Can you work these out from the drawing? Everything is in mm from the part's minimum corner. A direction names the side the tool comes from. Coordinates: 2 decimals unless noted, no trailing zeros. Order: outer loops, then holes, each group sorted by start corner. A loop starts at its lowest first (then second) coordinate and runs counter-clockwise, first axis right, second up. Notation, with made-up numbers: (-25.75, 22) -> (23.25, 22) arc R21 cw to (23.25, 47) -> close; hole circle Ø11 at (-6, -28). An arc over 180 degrees is marked (long way). Answer in a Markdown table with one row per item.
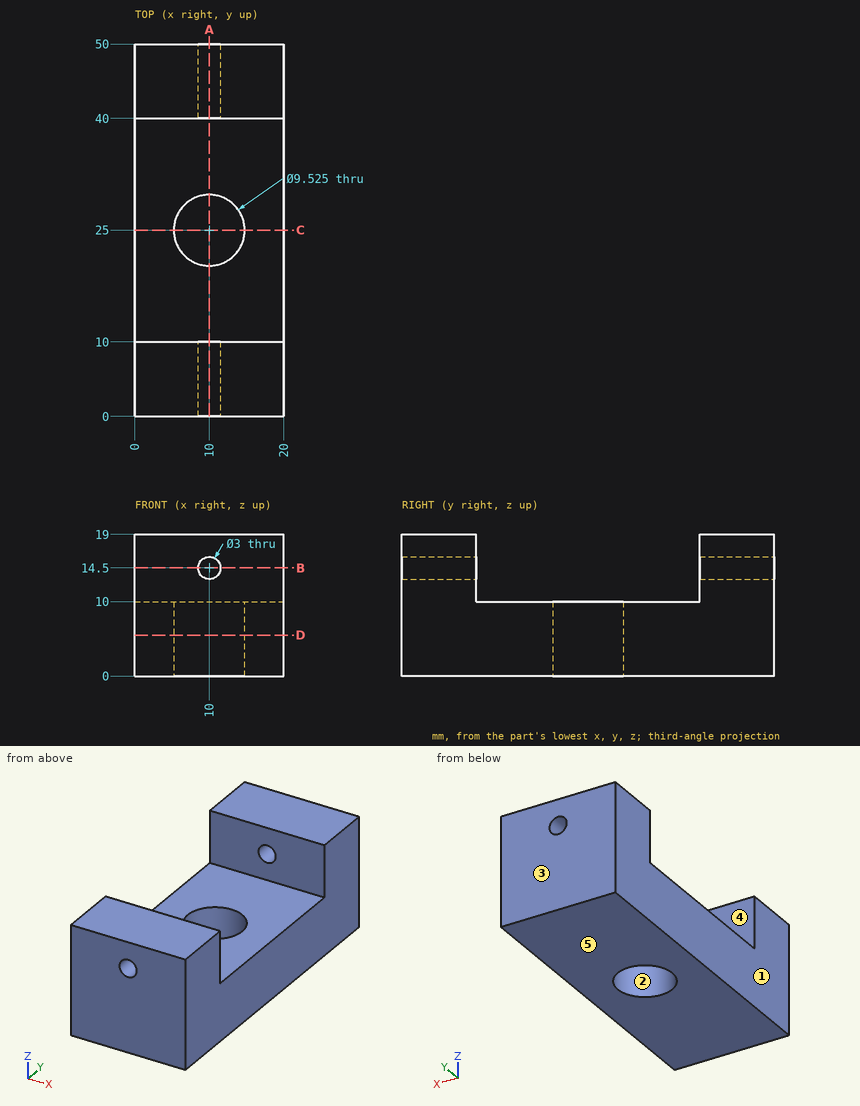
(1) We'd pull the mould along X, two halves only. Please class the marked faces 1, 2 and 3: +X half, -X half, draft (parallel to the pull), parting line (faces both ways), or undercut.
Response values:
| item | result |
|---|---|
| face 1 | -X half |
| face 2 | undercut |
| face 3 | draft |
(2) Suppose I cut it at B-B (z = 14.5). Please give me the cut outline in (x, y), and give its area (3 significant figures).
Response values:
| item | result |
|---|---|
| outline | (0, 0) -> (8.5, 0) -> (8.5, 10) -> (0, 10) -> close; (0, 40) -> (8.5, 40) -> (8.5, 50) -> (0, 50) -> close; (11.5, 0) -> (20, 0) -> (20, 10) -> (11.5, 10) -> close; (11.5, 40) -> (20, 40) -> (20, 50) -> (11.5, 50) -> close |
| area | 340 mm2 |
(3) Will this pin go through, and if not, where does the flat tip stop? pin 1 Ø12 at (x, y) = (3, 25) entering from +Z.
Response values:
| item | result |
|---|---|
| pin 1 | z = 10 |
(4) Suppose I cut it at A-A (x = 10). Please give me the cut outline in (y, z), and give its area (3 significant figures).
Response values:
| item | result |
|---|---|
| outline | (0, 0) -> (20.24, 0) -> (20.24, 10) -> (10, 10) -> (10, 13) -> (0, 13) -> close; (0, 16) -> (10, 16) -> (10, 19) -> (0, 19) -> close; (29.76, 0) -> (50, 0) -> (50, 13) -> (40, 13) -> (40, 10) -> (29.76, 10) -> close; (40, 16) -> (50, 16) -> (50, 19) -> (40, 19) -> close |
| area | 525 mm2 |
(5) On a 3-axis mill with a long thin cutter (end or side, diameter ignored), from which of +Z, -Z, +X, -X, +Y, -Y can I reach the whole of each face in a straight line? I mean the marked faces 4 and 5. Say none if no direction works.
Response values:
| item | result |
|---|---|
| face 4 | +Z, +X, -X |
| face 5 | -Z, +X, -X, +Y, -Y |
(6) Suppose I cut it at D-D (z = 5.5). Please give me the cut outline in (x, y) (1 decimal).
Response values:
| item | result |
|---|---|
| outline | (0, 0) -> (20, 0) -> (20, 50) -> (0, 50) -> close; hole circle Ø9.5 at (10, 25) |
(7) I need wall thicknesses on line 1 (Z direction, x = 10, y = 2.5); line 2 (X direction, y = 47.5, z = 14.5); line 3 (Y direction, x = 18, z = 13.75). Which ranges of each line are inside material? Lowest first, please. Write a range as [from, to].
Response values:
| item | result |
|---|---|
| line 1 | [0, 13], [16, 19] |
| line 2 | [0, 8.5], [11.5, 20] |
| line 3 | [0, 10], [40, 50] |
(8) Suppose I cut it at C-C (y = 25). Please give me the cut outline in (x, z), and give its area (3 significant figures).
Response values:
| item | result |
|---|---|
| outline | (0, 0) -> (5.24, 0) -> (5.24, 10) -> (0, 10) -> close; (14.76, 0) -> (20, 0) -> (20, 10) -> (14.76, 10) -> close |
| area | 105 mm2 |
